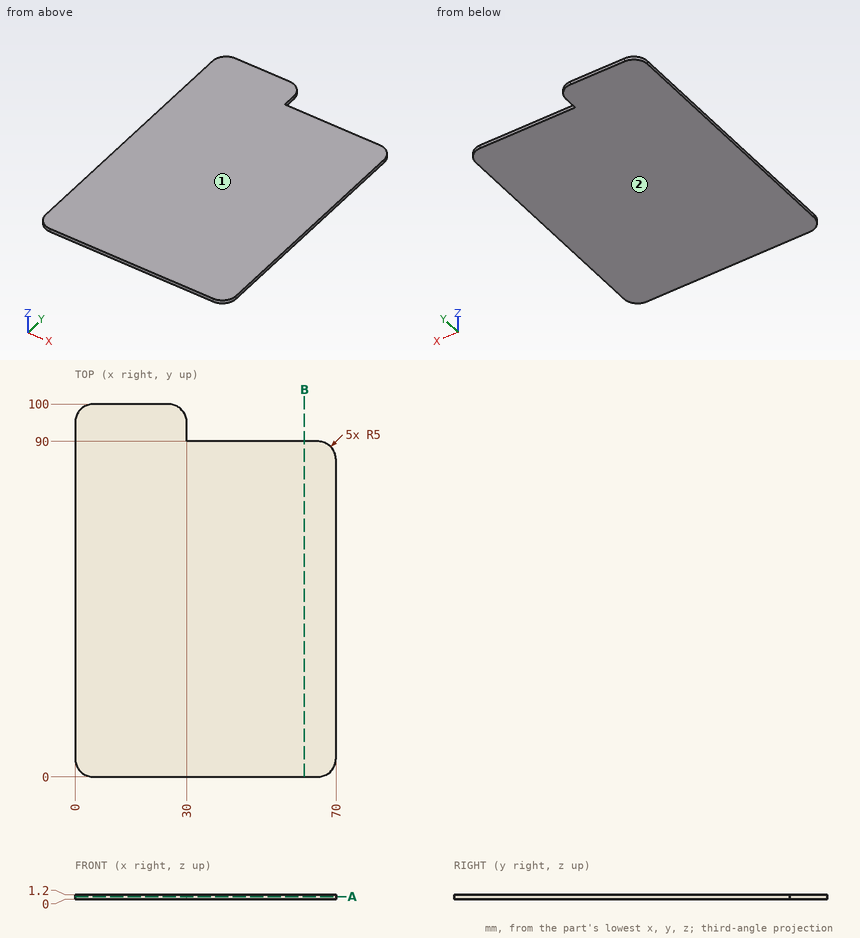
Source: three-view drawing plus pictorial views. Frame: mm from the lowest corner of the part. Coordinates: 2 decimals unless noted, no trailing zeros. Loops run counter-clockwise (first coordinate to the right, second up) from the corner with the lowest first, then second, coordinate; pieces in that order, holes last. Notation, with made-up numbers: (-30.75, 32.25) -> (10.25, 32.25) arc R13 cw to (10.25, 42.25) -> close; hole circle Ø6 at (59, 0.25). An arc over 180 degrees is marked (long way). Answer in a Markdown table with one row per item. Add a question column.
Q1. Section B-B on x = 61.5. Return the cut outline in (y, z), and give its area (3 significant figures).
Q2. Pull-direction query (Z, two-part tool) for the marked faces 1 and 2; classes: pulls with the +Z half, pulls with the -Z half, needs draft (parallel to the pull), parting line crosses it, or undercut.
Q3. Section A-A on z = 0.75. Return the cut outline in (x, y), and give its area (3 significant figures).
Q4. Ray query, line 1 along Y through (x, z) = (47.5, 0.65); line 2 along X through (y, z) = (4, 0.3); line 3 along X through (y, z) = (89, 0.75). Return the intervals inside material, ascending.
Q5. Contact query for a flat-ended pin moving along its axis: pin 1 Ø0.6 at (x, z) = (41.5, 0.5) entering from +Y. Output: stop coordinate, or through.
Computed values:
| question | item | result |
|---|---|---|
| 1 | outline | (0, 0) -> (90, 0) -> (90, 1.2) -> (0, 1.2) -> close |
| 1 | area | 108 mm^2 |
| 2 | face 1 | pulls with the +Z half |
| 2 | face 2 | pulls with the -Z half |
| 3 | outline | (0, 5) arc R5 ccw to (5, 0) -> (65, 0) arc R5 ccw to (70, 5) -> (70, 85) arc R5 ccw to (65, 90) -> (30, 90) -> (30, 95) arc R5 ccw to (25, 100) -> (5, 100) arc R5 ccw to (0, 95) -> close |
| 3 | area | 6,570 mm^2 |
| 4 | line 1 | y = 0 to 90 |
| 4 | line 2 | x = 0.1 to 69.9 |
| 4 | line 3 | x = 0 to 68 |
| 5 | pin 1 | stops at y = 90 |
